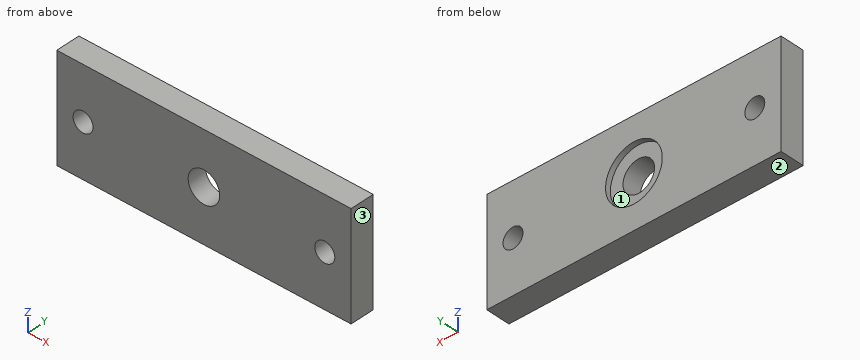
Autodesk Inventor part; units mm, degrees
ref_plane "YZ Plane" through (0, 0, 0) normal (1, 0, 0) x (0, 1, 0)
ref_plane "XZ Plane" through (0, 0, 0) normal (0, 1, 0) x (-1, 0, 0)
ref_plane "XY Plane" through (0, 0, 0) normal (0, 0, 1) x (1, 0, 0)
sketch "Sketch2" plane through (0, 0, 0) normal (0, 1, 0) x (-1, 0, 0)
  line L0 (0, 0) -> (280, 0)
  line L1 (280, 0) -> (280, -100)
  line L2 (280, -100) -> (0, -100)
  line L3 (0, -100) -> (0, 0)
  circle A0 centre (140, -50) radius 15
  circle A1 centre (255, -50) radius 9.5
  circle A2 centre (25, -50) radius 9.5
  dimension "d0" = 280
  dimension "d1" = 100
  dimension "d2" = 30
  dimension "d3" = 19
  dimension "d4" = 19
  dimension "d5" = 115
  dimension "d6" = 115
extrude "Extrusion2" add sketch "Sketch2" along normal blind 23
sketch "Sketch4" plane through (0, 23, 0) normal (0, 1, 0) x (1, 0, 0)
  circle A0 centre (-140, 50) radius 27
  point P0 (0, 0)
  dimension "d11" = 54
extrude "Extrusion3" cut sketch "Sketch4" against normal blind 5
sketch "Sketch5" plane through (0, 23, 0) normal (0, 1, 0) x (1, 0, 0)
  point P0 (0, 0)
properties part number "top plate"
Here's how the part is built. I have some questions about the finished solid (model axes, mm). Face numbers are marked on the shaded views. Give positions to 0.01 mm unless a question says otherwise; leave off trailing zeros. Write each loop counter-clockwise with the first axis right and the second up, starting at its lowest first coordinate (ties: lowest second). Pieces come first, ordered by that corner, then holes. Notation, with made-up numbers: (51.25, 48) -> (93.25, 48) arc R20 ccw to (93.25, 81) -> close; hole circle Ø7 at (12, -6.75). An arc over 180 degrees is marked (long way). Write each question's results on one line, items separated by ' | '.
Item 1: If I drill on L1, parallel to Z at x = -140, y = 20.6; L2, parallel to X at y = 20, z = -50.5; L3, parallel to X at y = 7, z = -51.5, over which ranges is the centre line in solid material (lowest first)?
Output:
L1: z = -100 to -77, -23 to 0 | L2: x = -280 to -264.49, -245.51 to -167, -113 to -34.49, -15.51 to 0 | L3: x = -280 to -264.38, -245.62 to -154.92, -125.08 to -34.38, -15.62 to 0
Item 2: Suppose I cut it at B-B on z = -50. Write out the boundary of the cut face in (x, y), plus the area to 3 significant figures.
Output:
outline: (-280, 0) -> (-264.5, 0) -> (-264.5, 23) -> (-280, 23) -> close; (-245.5, 0) -> (-155, 0) -> (-155, 18) -> (-167, 18) -> (-167, 23) -> (-245.5, 23) -> close; (-125, 0) -> (-34.5, 0) -> (-34.5, 23) -> (-113, 23) -> (-113, 18) -> (-125, 18) -> close; (-15.5, 0) -> (0, 0) -> (0, 23) -> (-15.5, 23) -> close | area: 4,760 mm^2
Item 3: Suppose I cut it at A-A on x = -140. Write out the boundary of the cut face in (y, z), plus the area to 3 significant figures.
Output:
outline: (0, -100) -> (23, -100) -> (23, -77) -> (18, -77) -> (18, -65) -> (0, -65) -> close; (0, -35) -> (18, -35) -> (18, -23) -> (23, -23) -> (23, 0) -> (0, 0) -> close | area: 1,490 mm^2
Item 4: Suppose I cut it at C-C on y = 4.5. Write out the boundary of the cut face in (x, z).
Output:
outline: (-280, -100) -> (0, -100) -> (0, 0) -> (-280, 0) -> close; hole circle Ø19 at (-255, -50); hole circle Ø30 at (-140, -50); hole circle Ø19 at (-25, -50)
Item 5: Suppose I cut it at D-D on x = -25. Write out the boundary of the cut face in (y, z).
Output:
outline: (0, -100) -> (23, -100) -> (23, -59.5) -> (0, -59.5) -> close; (0, -40.5) -> (23, -40.5) -> (23, 0) -> (0, 0) -> close
Item 6: We'd pull the mould along X, two halves only. Please class the marked faces 1, 2 and 3: pulls with the +X half, pulls with the -X half, needs draft (parallel to the pull), parting line crosses it, or undercut.
Output:
face 1: undercut | face 2: needs draft | face 3: pulls with the +X half
